Input: part model. Units: mm. Frame: model coordinates. A direction names the side the tool comes from. Round coordinates to 2 decimals unless told otherwise and drop trailing zeros. Order: outer loops, then holes, each group sorted by start corner. A loop starts at its lowest first (then second) coordinate and runs counter-clockwise, first axis right, second up.
Item 1: Cut plane B-B on y = -1.45. Give the number of separate pieces and of enclosed holes in the cut face, then the cut area to 3 significant figures.
Item 2: Reachability of faces 4 (the flat face through (0, -2.794, 8)), 5 (the flat face through (11.985, 1, 8)) from +Z, -Z, +X, -X, +Y, -Y: full face, straight path, thin tool, end or side. Return the list, or none.
Item 3: Line query: L1, parallel to Y at x = -10, z = 13.5. Output: solid intervals per line, ascending.
Item 4: Cut plane A-A on x = -10. Output: boundary loops of the cut face in (y, z), then the cut area to 3 significant figures.
Item 5: Mould query, pull axis X, two halves, no side actions, for faces 1 (the flat face through (-16.51, 0, 8)), 2 (the flat face through (0, 0, 0)), 3 (the flat face through (-14.525, -1, 8)). Classes: released by +X, released by -X, zero draft, split by the parting line, or undercut.
```python
from build123d import *

# Parameters (mm, degrees)
SKETCH1_W           = 33.02
SKETCH1_H           = 5.588
SKETCH1_W_2         = 1.397
SKETCH1_H_2         = 1.397
SKETCH1_W_3         = 1.364533422
BOSS_EXTRUDE1_DEPTH = 15.24


with BuildPart() as part:
    # Sketch1 → Boss-Extrude1 (new body)
    with BuildSketch(Plane.XY):
        Rectangle(SKETCH1_W, SKETCH1_H)
        with Locations((2.523766711, -1.451626982)):
            Rectangle(SKETCH1_W_2, SKETCH1_H_2, mode=Mode.SUBTRACT)
        with Locations((0, -1.451626982)):
            Rectangle(SKETCH1_W_3, SKETCH1_H_2, mode=Mode.SUBTRACT)
        with Locations((5.063766711, -1.451626982)):
            Rectangle(SKETCH1_W_2, SKETCH1_H_2, mode=Mode.SUBTRACT)
        with Locations((7.603766711, -1.451626982)):
            Rectangle(SKETCH1_W_2, SKETCH1_H_2, mode=Mode.SUBTRACT)
        with Locations((10.143766711, -1.451626982)):
            Rectangle(SKETCH1_W_2, SKETCH1_H_2, mode=Mode.SUBTRACT)
        with Locations((12.683766711, -1.451626982)):
            Rectangle(SKETCH1_W_2, SKETCH1_H_2, mode=Mode.SUBTRACT)
        with Locations((15.223766711, -1.451626982)):
            Rectangle(SKETCH1_W_2, SKETCH1_H_2, mode=Mode.SUBTRACT)
        with Locations((-15.223766711, -1.451626982)):
            Rectangle(SKETCH1_W_2, SKETCH1_H_2, mode=Mode.SUBTRACT)
        with Locations((-12.683766711, -1.451626982)):
            Rectangle(SKETCH1_W_2, SKETCH1_H_2, mode=Mode.SUBTRACT)
        with Locations((-10.143766711, -1.451626982)):
            Rectangle(SKETCH1_W_2, SKETCH1_H_2, mode=Mode.SUBTRACT)
        with Locations((-7.603766711, -1.451626982)):
            Rectangle(SKETCH1_W_2, SKETCH1_H_2, mode=Mode.SUBTRACT)
        with Locations((-5.063766711, -1.451626982)):
            Rectangle(SKETCH1_W_2, SKETCH1_H_2, mode=Mode.SUBTRACT)
        with Locations((-2.523766711, -1.451626982)):
            Rectangle(SKETCH1_W_2, SKETCH1_H_2, mode=Mode.SUBTRACT)
        with Locations((-2.523766711, 1.451626982)):
            Rectangle(SKETCH1_W_2, SKETCH1_H_2, mode=Mode.SUBTRACT)
        with Locations((0, 1.451626982)):
            Rectangle(SKETCH1_W_3, SKETCH1_H_2, mode=Mode.SUBTRACT)
        with Locations((-5.063766711, 1.451626982)):
            Rectangle(SKETCH1_W_2, SKETCH1_H_2, mode=Mode.SUBTRACT)
        with Locations((-7.603766711, 1.451626982)):
            Rectangle(SKETCH1_W_2, SKETCH1_H_2, mode=Mode.SUBTRACT)
        with Locations((-10.143766711, 1.451626982)):
            Rectangle(SKETCH1_W_2, SKETCH1_H_2, mode=Mode.SUBTRACT)
        with Locations((-12.683766711, 1.451626982)):
            Rectangle(SKETCH1_W_2, SKETCH1_H_2, mode=Mode.SUBTRACT)
        with Locations((-15.223766711, 1.451626982)):
            Rectangle(SKETCH1_W_2, SKETCH1_H_2, mode=Mode.SUBTRACT)
        with Locations((15.223766711, 1.451626982)):
            Rectangle(SKETCH1_W_2, SKETCH1_H_2, mode=Mode.SUBTRACT)
        with Locations((12.683766711, 1.451626982)):
            Rectangle(SKETCH1_W_2, SKETCH1_H_2, mode=Mode.SUBTRACT)
        with Locations((10.143766711, 1.451626982)):
            Rectangle(SKETCH1_W_2, SKETCH1_H_2, mode=Mode.SUBTRACT)
        with Locations((7.603766711, 1.451626982)):
            Rectangle(SKETCH1_W_2, SKETCH1_H_2, mode=Mode.SUBTRACT)
        with Locations((5.063766711, 1.451626982)):
            Rectangle(SKETCH1_W_2, SKETCH1_H_2, mode=Mode.SUBTRACT)
        with Locations((2.523766711, 1.451626982)):
            Rectangle(SKETCH1_W_2, SKETCH1_H_2, mode=Mode.SUBTRACT)
    extrude(amount=BOSS_EXTRUDE1_DEPTH)


solid = part.part
```
From the geometry:
1. separate pieces: 14
1. enclosed holes: 0
1. area: 227 mm2
2. face 4: +Z, -Z, +X, -X, -Y
2. face 5: +Z, -Z
3. L1: y = -2.79 to -2.15, -0.75 to 0.75, 2.15 to 2.79
4. outline: (-2.79, 0) - (-2.15, 0) - (-2.15, 15.24) - (-2.79, 15.24) - close; (-0.75, 0) - (0.75, 0) - (0.75, 15.24) - (-0.75, 15.24) - close; (2.15, 0) - (2.79, 0) - (2.79, 15.24) - (2.15, 15.24) - close
4. area: 42.6 mm2
5. face 1: released by -X
5. face 2: zero draft
5. face 3: undercut
